For this review, take the finished solid that the model builds, in its own axes (mm). Face numbers are marked on the shaded views. A direction names the side the tool comes from. Coordinates: 2 decimals unless noted, no trailing zeros. Loops run counter-clockwise (first coordinate to the right, second up) from the corner with the lowest first, then second, coordinate; pieces in that order, holes last. Notation, with made-up numbers: (20.25, 74.5) -> (29.25, 74.5) arc R6 ccw to (29.25, 83.5) -> close; hole circle Ø6 at (-26, 73). An arc over 180 degrees is marked (long way). Answer in a Markdown table with one row per item.
from build123d import *

# Parameters (mm, degrees)
F0_W      = 25.4
F0_H      = 25.4
F1_DEPTH  = 25.4
F2_R      = 5.08
F3_DEPTH  = 2.54
F4_DEPTH  = 2.54
F5_DEPTH  = 2.54
F6_DEPTH  = 2.54
F7_DEPTH  = 2.54
F8_DEPTH  = 2.54
F15_DEPTH = 2.54
F11_W     = 7.62
F11_H     = 7.62
F16_DEPTH = 2.54
F17_DEPTH = 2.54
F18_DEPTH = 2.54
F19_DEPTH = 2.54
F20_DEPTH = 2.54


with BuildPart() as f1:
    # F0 (on Front) → F1 (new body)
    with BuildSketch(Plane.XZ):
        with Locations((12.7, 12.7)):
            Rectangle(F0_W, F0_H)
    extrude(amount=F1_DEPTH)

    # F2
    f2_edges = [f1.edges().sort_by_distance(p)[0] for p in [
        (12.7, -25.4, 25.4),
        (12.7, -25.4, 0),
        (12.7, 0, 25.4),
        (12.7, 0, 0),
        (25.4, 0, 12.7),
        (0, 0, 12.7),
        (0, -12.7, 25.4),
        (0, -12.7, 0),
        (25.4, -12.7, 25.4),
        (25.4, -25.4, 12.7),
        (0, -25.4, 12.7),
        (25.4, -12.7, 0),
    ]]
    fillet(f2_edges, radius=F2_R)

    # F3 (cut): a face of the model
    f3_faces = [f1.faces().sort_by_distance(p)[0] for p in [
        (12.7, -25.4, 12.7),
    ]]
    extrude(f3_faces, amount=-F3_DEPTH, mode=Mode.SUBTRACT)

    # F4 (cut): a face of the model
    f4_faces = [f1.faces().sort_by_distance(p)[0] for p in [
        (0, -12.7, 12.7),
    ]]
    extrude(f4_faces, amount=-F4_DEPTH, mode=Mode.SUBTRACT)

    # F5 (cut): a face of the model
    f5_faces = [f1.faces().sort_by_distance(p)[0] for p in [
        (12.7, -12.7, 25.4),
    ]]
    extrude(f5_faces, amount=-F5_DEPTH, mode=Mode.SUBTRACT)

    # F6 (cut): a face of the model
    f6_faces = [f1.faces().sort_by_distance(p)[0] for p in [
        (25.4, -12.7, 12.7),
    ]]
    extrude(f6_faces, amount=-F6_DEPTH, mode=Mode.SUBTRACT)

    # F7 (cut): a face of the model
    f7_faces = [f1.faces().sort_by_distance(p)[0] for p in [
        (12.7, -12.7, 0),
    ]]
    extrude(f7_faces, amount=-F7_DEPTH, mode=Mode.SUBTRACT)

    # F8 (cut): a face of the model
    f8_faces = [f1.faces().sort_by_distance(p)[0] for p in [
        (12.7, 0, 12.7),
    ]]
    extrude(f8_faces, amount=-F8_DEPTH, mode=Mode.SUBTRACT)

    # F14 (on face) → F15 (join)
    with BuildSketch(Plane.XY.offset(22.86)):
        Polygon((20.32, -20.32), (20.32, -12.7), (5.08, -5.08), (5.08, -12.7), align=None)
    extrude(amount=F15_DEPTH)

    # F11 (on face) → F16 (join)
    with BuildSketch(Plane(origin=(0, -2.54, 0), x_dir=(-1, 0, 0), z_dir=(0, 1, 0))):
        with Locations((-12.7, 12.7)):
            Rectangle(F11_W, F11_H)
    extrude(amount=F16_DEPTH)

    # F9 (on face) → F17 (join)
    with BuildSketch(Plane.XZ.offset(22.86)):
        Polygon((12.7, 5.08), (5.08, 12.7), (5.08, 5.08), align=None)
        Polygon((12.7, 20.32), (5.08, 12.7), (12.7, 5.08), (20.32, 12.7), align=None)
        Polygon((20.32, 20.32), (12.7, 20.32), (20.32, 12.7), align=None)
    extrude(amount=F17_DEPTH)

    # F12 (on face) → F18 (join)
    with BuildSketch(Plane(origin=(2.54, 0, 0), x_dir=(0, -1, 0), z_dir=(-1, 0, 0))):
        Polygon((16.51, 20.32), (12.7, 20.32), (8.89, 20.32), (8.89, 16.51), (5.08, 16.51), (5.08, 12.7), (5.08, 8.89), (8.89, 8.89), (8.89, 5.08), (12.7, 5.08), (16.51, 5.08), (16.51, 8.89), (20.32, 8.89), (20.32, 12.7), (20.32, 16.51), (16.51, 16.51), align=None)
    extrude(amount=F18_DEPTH)

    # F13 (on face) → F19 (join)
    with BuildSketch(Plane(origin=(0, 0, 2.54), x_dir=(1, 0, 0), z_dir=(0, 0, -1))):
        Polygon((12.7, 8.89), (20.32, 5.08), (20.32, 20.32), (12.7, 16.51), (5.08, 12.7), align=None)
        Polygon((5.08, 5.08), (12.7, 8.89), (5.08, 12.7), align=None)
        Polygon((5.08, 20.32), (5.08, 12.7), (12.7, 16.51), align=None)
    extrude(amount=F19_DEPTH)

    # F10 (on face) → F20 (join)
    with BuildSketch(Plane.YZ.offset(22.86)):
        with BuildLine():
            Line((-5.08, 5.08), (-5.08, 12.7))
            ThreePointArc((-5.08, 12.7), (-7.3118463274, 7.3118463274), (-12.7, 5.08))
            Line((-12.7, 5.08), (-5.08, 5.08))
        make_face()
        with BuildLine():
            ThreePointArc((-12.7, 20.32), (-7.3118463274, 18.0881536726), (-5.08, 12.7))
            Line((-5.08, 12.7), (-5.08, 20.32))
            Line((-5.08, 20.32), (-12.7, 20.32))
        make_face()
        with BuildLine():
            ThreePointArc((-20.32, 12.7), (-18.0881536726, 18.0881536726), (-12.7, 20.32))
            Line((-12.7, 20.32), (-20.32, 20.32))
            Line((-20.32, 20.32), (-20.32, 12.7))
        make_face()
        with BuildLine():
            Line((-20.32, 5.08), (-12.7, 5.08))
            ThreePointArc((-12.7, 5.08), (-18.0881536726, 7.3118463274), (-20.32, 12.7))
            Line((-20.32, 12.7), (-20.32, 5.08))
        make_face()
    extrude(amount=F20_DEPTH)


solid = f1.part
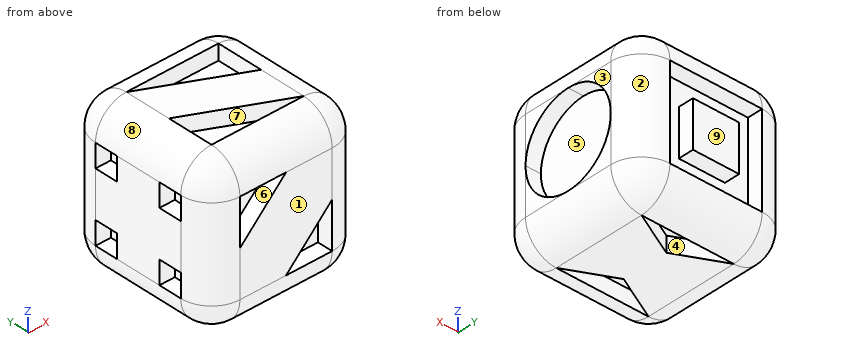
Item 1: For the marked faces 5, 6, 7, 8 and 9, list the 3-axis set-ups (+Z, -Z, +X, -X, +Y, -Y) from which the entire face can be reached by the end or side of a thin tool; tool diameter is ignored.
Worked answers:
| item | result |
|---|---|
| face 5 | +X |
| face 6 | -Y |
| face 7 | +Z |
| face 8 | +Z, -X, +Y, -Y |
| face 9 | +Z, -Z, +X, -X, +Y |
Item 2: The part is to be moulded in two halves that separate along Y. For the marked faces 1, 2, 3 and 4, say which applies: +Y half, -Y half, draft (parallel to the pull), parting line (faces both ways), or undercut.
Worked answers:
| item | result |
|---|---|
| face 1 | -Y half |
| face 2 | +Y half |
| face 3 | draft |
| face 4 | undercut |
Item 3: Take a section at C-C, the plane x = 24. State the section outline as (y, z) points.
Worked answers:
| item | result |
|---|---|
| outline | (-23.82, 5.08) arc R3.5 ccw to (-20.32, 1.58) -> (-5.08, 1.58) arc R3.5 ccw to (-1.58, 5.08) -> (-1.58, 20.32) arc R3.5 ccw to (-5.08, 23.82) -> (-20.32, 23.82) arc R3.5 ccw to (-23.82, 20.32) -> close; hole circle Ø15.24 at (-12.7, 12.7) |
Item 4: Insertion check: pin 1 (1.3 mm diameter, centred on x = 15.5, y = -24.5, fed in from +Z); pin 2 (3 mm diameter, centred on y = -24, z = 18, fed in from +X); pin 3 (2 mm diameter, centred on x = 1, z = 18, fed in from +Y). Each pin has a flat end and moves straight along its axis. Give the tip position at first contact, or say it passes through.
Worked answers:
| item | result |
|---|---|
| pin 1 | z = 23.97 |
| pin 2 | x = 24.91 |
| pin 3 | y = -1.04 |
Item 5: For L1, parallel to Y at x = 13.75, z = 24.5 (3 decimals); L2, parallel to Z at x = 12.5, y = -1; L3, parallel to Z at x = 15.75, y = -10.25, list the stretches that pass through material, from the lowest coordinate up.
Worked answers:
| item | result |
|---|---|
| L1 | -23.207 to -20.32, -17.035 to -9.415, -5.08 to -2.193 |
| L2 | 2.05 to 5.08, 8.89 to 16.51, 20.32 to 23.35 |
| L3 | 0 to 22.86 |
Item 6: Take a section at B-B, the plane y = -21.25. State the section outline as (x, z) points.
Worked answers:
| item | result |
|---|---|
| outline | (0.09, 5.08) arc R4.99 ccw to (5.08, 0.09) -> (20.32, 0.09) arc R4.99 ccw to (25.31, 5.08) -> (25.31, 20.32) arc R4.99 ccw to (20.32, 25.31) -> (5.08, 25.31) arc R4.99 ccw to (0.09, 20.32) -> close |
Item 7: Take a section at A-A, the plane z = 21.5. State the section outline as (x, y) points, and give its area (3 significant figures).
Worked answers:
| item | result |
|---|---|
| outline | (0.14, -20.32) arc R4.94 ccw to (5.08, -25.26) -> (20.32, -25.26) arc R4.94 ccw to (25.26, -20.32) -> (25.26, -5.08) arc R4.94 ccw to (20.32, -0.14) -> (5.08, -0.14) arc R4.94 ccw to (0.14, -5.08) -> close |
| area | 610 mm² |
